from build123d import *

# Parameters (mm, degrees)
EXTRUDE_1_DEPTH = 6
SKETCH_2_R      = 1.25
EXTRUDE_2_DEPTH = 2
SKETCH_3_R      = 1
EXTRUDE_4_DEPTH = 1.75
SKETCH_4_R      = 1
EXTRUDE_7_DEPTH = 1.75


with BuildPart() as part:
    # 스케치1 → 보스-돌출1 (new body)
    with BuildSketch(Plane.XY):
        Polygon((0, 4.618802154), (-4, 2.309401077), (-4, -2.309401077), (0, -4.618802154), (4, -2.309401077), (4, 2.309401077), align=None)
        Polygon((0, 2.598076211), (-2.25, 1.299038106), (-2.25, -1.299038106), (0, -2.598076211), (2.25, -1.299038106), (2.25, 1.299038106), align=None, mode=Mode.SUBTRACT)
    extrude(amount=EXTRUDE_1_DEPTH)

    # 스케치2 → 보스-돌출2 (add)
    with BuildSketch(Plane(origin=(0, 0, 0), x_dir=(-1, 0, 0), z_dir=(0, 0, -1))):
        Polygon((0, 4.618802154), (-4, 2.309401077), (-4, -2.309401077), (0, -4.618802154), (4, -2.309401077), (4, 2.309401077), align=None)
        Circle(SKETCH_2_R, mode=Mode.SUBTRACT)
    extrude(amount=EXTRUDE_2_DEPTH)

    # 스케치3 → 보스-돌출4 (add)
    with BuildSketch(Plane(origin=(2, 3.464101615, 0), x_dir=(0.866025404, -0.5, 0), z_dir=(0.5, 0.866025404, 0))):
        with BuildLine():
            Line((-2.309401077, -6), (2.309401077, -6))
            Line((2.309401077, -6), (2.309401077, -10))
            ThreePointArc((2.309401077, -10), (0, -12.309401077), (-2.309401077, -10))
            Line((-2.309401077, -10), (-2.309401077, -6))
        make_face()
        with Locations((0, -10)):
            Circle(SKETCH_3_R, mode=Mode.SUBTRACT)
    extrude(amount=-EXTRUDE_4_DEPTH)

    # 스케치4 → 보스-돌출7 (add)
    with BuildSketch(Plane(origin=(-2, -3.464101615, 0), x_dir=(0.866025404, -0.5, 0), z_dir=(-0.5, -0.866025404, 0))):
        with BuildLine():
            Line((-2.309401077, 10), (-2.309401077, 6))
            Line((-2.309401077, 6), (2.309401077, 6))
            Line((2.309401077, 6), (2.309401077, 10))
            ThreePointArc((2.309401077, 10), (0, 12.309401077), (-2.309401077, 10))
        make_face()
        with Locations((0, 10)):
            Circle(SKETCH_4_R, mode=Mode.SUBTRACT)
    extrude(amount=-EXTRUDE_7_DEPTH)


solid = part.part
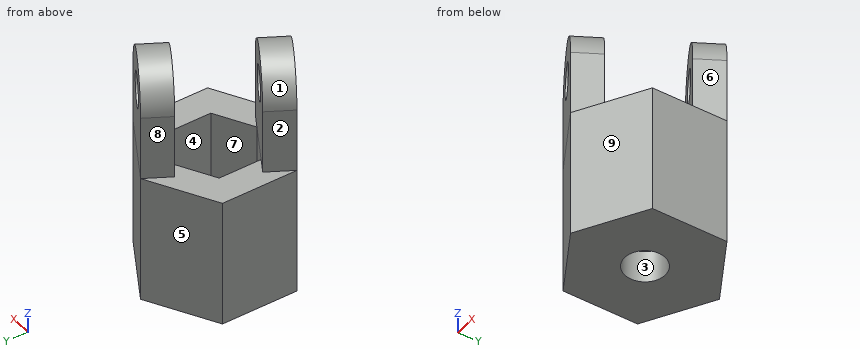
For this review, take the finished solid that the model builds, in its own axes (mm). Face numbers are marked on the shaded views. A direction names the side the tool comes from. Round coordinates to 2 decimals unless told otherwise and drop trailing zeros. Order: outer loops, then holes, each group sorted by start corner. A loop starts at its lowest first (then second) coordinate and runs counter-clockwise, first axis right, second up. Notation, with made-up numbers: (-9.5, 61) -> (41.5, 61) arc R14 cw to (41.5, 85) -> close; hole circle Ø8 at (88.25, 50). An arc over 180 degrees is marked (long way). Write item = value, one per line. Start each with the question number.
1) The part is to be moulded in two halves that separate along X. For the marked faces 1, 2, 3 and 4, say which applies: +X half, -X half, draft (parallel to the pull), parting line (faces both ways), or undercut.
2) Take a section at B-B on y = 0. State the section outline as (x, z) points.
3) Take a section at C-C on z = 6.75. State the section outline as (x, y) points (3 decimals).
4) To check wall thickness, follow line 1 (X direction, y = -0.5, z = 2); line 2 (Z direction, x = -2.5, y = 2); line 3 (Z direction, x = -1.5, y = 0.5). State the ranges of each line that lie inside material, in increasing order. Write a range as from..to.
5) Tool access review of the marked faces 5, 6, 7, 8 and 9: name each direction out of +Z, -Z, +X, -X, +Y, -Y from which nothing blocks a thin tool from reaching the whole face with its end or side.
6) Insertion check: pin 1 (1.3 mm diameter, centred on x = 0.5, y = -1, fed in from +Z); pin 2 (3 mm diameter, centred on x = 2.5, y = -1.5, fed in from +Z); pin 3 (1 mm diameter, centred on x = -2, z = 1.5, fed in from +Y). Each pin has a flat end and moves straight along its axis. Give the tip position at first contact, or say it passes through.
7) Take a section at D-D on z = 10.25. State the section outline as (x, y) points.
8) Take a section at A-A on z = 0.5. State the section outline as (x, y) points, plus the area to 3 significant figures.
Verdict:
q1.face_1 = parting line
q1.face_2 = -X half
q1.face_3 = undercut
q1.face_4 = undercut
q2.outline = (-4, -2) -> (-1.25, -2) -> (-1.25, 0) -> (-2.25, 0) -> (-2.25, 6) -> (-4, 6) -> close; (1.25, -2) -> (4, -2) -> (4, 6) -> (2.25, 6) -> (2.25, 0) -> (1.25, 0) -> close
q3.outline = (-4, -2.309) -> (0, -4.619) -> (0.875, -3.103) -> (-3.125, -0.794) -> close; (-0.875, 3.103) -> (3.125, 0.794) -> (4, 2.309) -> (0, 4.619) -> close
q4.line_1 = -4..-2.25, 2.25..4
q4.line_2 = -2..6
q4.line_3 = -2..0
q5.face_5 = +Z, -Z, -X, +Y
q5.face_6 = +Z, +X, -Y
q5.face_7 = +Z
q5.face_8 = +Z, -X, +Y
q5.face_9 = +Z, -Z, +X, -Y
q6.pin_1 = 0
q6.pin_2 = 6
q6.pin_3 = 3.75
q7.outline = (-3.99, -2.32) -> (-2.84, -2.98) -> (-1.96, -1.46) -> (-3.11, -0.8) -> close; (-1.16, -3.95) -> (-0.01, -4.61) -> (0.86, -3.1) -> (-0.29, -2.43) -> close; (-0.86, 3.1) -> (0.29, 2.43) -> (1.16, 3.95) -> (0.01, 4.61) -> close; (1.96, 1.46) -> (3.11, 0.8) -> (3.99, 2.32) -> (2.84, 2.98) -> close
q8.outline = (-4, -2.31) -> (0, -4.62) -> (4, -2.31) -> (4, 2.31) -> (0, 4.62) -> (-4, 2.31) -> close; hole (-2.25, -1.3) -> (0, -2.6) -> (2.25, -1.3) -> (2.25, 1.3) -> (0, 2.6) -> (-2.25, 1.3) -> close
q8.area = 37.9 mm2
